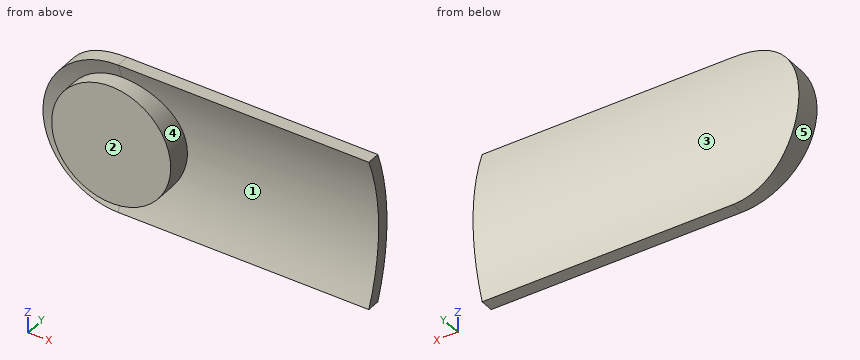
from build123d import *

# Parameters (mm, degrees)
F0_R     = 60.325
F1_DEPTH = 19.05
F4_ANGLE = -180
F2_R     = 203.2
F5_DEPTH = 492.64856
F6_DEPTH = 285.85777
F7_DEPTH = 25.4


with BuildPart() as f1:
    # F0 (on Front) → F1 (new body, symmetric)
    with BuildSketch(Plane.XZ):
        with BuildLine():
            Line((254, 76.2), (0, 76.2))
            ThreePointArc((0, 76.2), (-76.2, 0), (0, -76.2))
            Line((0, -76.2), (254, -76.2))
            Line((254, -76.2), (254, 76.2))
        make_face()
        Circle(F0_R, mode=Mode.SUBTRACT)
        Circle(F0_R)
    extrude(amount=F1_DEPTH, both=True)

    # F3 (on face) → F4 (revolve, cut)
    with BuildSketch(Plane.YZ):
        with BuildLine():
            Line((-406.4, 0), (0, 0))
            ThreePointArc((0, 0), (-203.2, 203.2), (-406.4, 0))
        make_face()
    revolve(axis=Axis((0, -203.2, 0), (0, 1, 0)), revolution_arc=F4_ANGLE, mode=Mode.SUBTRACT)

    # F2 (on Right) → F5 (cut)
    with BuildSketch(Plane.YZ):
        with Locations((-203.2, 0)):
            Circle(F2_R)
    extrude(amount=F5_DEPTH, mode=Mode.SUBTRACT)

    # F2 (on Right) → F6 (cut, symmetric)
    with BuildSketch(Plane.YZ):
        with BuildLine():
            ThreePointArc((-13.238437, 102.60319), (12.640691, -5.060247), (-18.255432, -111.392625))
            Line((-18.255432, -111.392625), (114.283874, -111.392625))
            Line((114.283874, -111.392625), (114.283874, 102.60319))
            Line((114.283874, 102.60319), (-13.238437, 102.60319))
        make_face()
    extrude(amount=F6_DEPTH, both=True, mode=Mode.SUBTRACT)

    # F0 (on Front) → F7 (join)
    with BuildSketch(Plane.XZ):
        Circle(F0_R)
    extrude(amount=F7_DEPTH)


solid = f1.part
Build history of the part. All positions in model axes, mm. Face numbers are marked on the shaded views. A direction names the side the tool comes from. Coordinates: 2 decimals unless noted, no trailing zeros. Write each loop counter-clockwise with the first axis right and the second up, starting at its lowest first coordinate (ties: lowest second). Pieces come first, ordered by that corner, then holes.
(1) 3-axis set-ups, long thin cutter, end or side, ignore diameter. For the marked faces 4 and 5: which of +Z, -Z, +X, -X, +Y, -Y reach the whole face in a straight line?
(2) Cut at B-B on x = 39.5. List the corners of the cut face in (y, z), and give its area (3 significant figures).
(3) Pin check, flat tips, straight feed: pin 1 Ø4 at (x, z) = (205.5, 49) entering from +Y; pin 2 Ø2 at (x, z) = (161.5, -38.5) entering from -Y; pin 3 Ø1 at (x, z) = (5.5, -42) entering from +Y. Stop position of each tip, or through.
(4) Mould opens along Z. For the marked faces 1, 2 and 3 say: pulls with the +Z half, pulls with the -Z half, needs draft (parallel to the pull), parting line crosses it, or undercut.
(5) Cut at D-D on x = 196. List the corners of the cut face in (y, z).
(6) Drill centre lines: line 1 (X direction, y = -4, z = 0.5); line 2 (Y direction, x = -45.5, z = 4.5); line 3 (Y direction, x = 27, z = -6). Where is each one in solid material? Low to high.
(7) Cut at C-C on y = -21. List the corners of the cut face in (x, z) (3 decimals), and give its area (3 significant figures).
(8) Cut at A-A on z = 0. List the corners of the cut face in (x, y) (3 decimals).
Working result:
1. face 4: -Y
1. face 5: -X, +Y, -Y
2. outline: (-25.4, -45.59) - (-5.18, -45.59) arc R203.2 cw to (-14.83, -76.2) - (-1.19, -76.2) arc R215.9 ccw to (-1.19, 76.2) - (-14.83, 76.2) arc R203.2 cw to (-5.18, 45.59) - (-25.4, 45.59) - close
2. area: 4,140 mm2
3. pin 1: stops at y = 7.52
3. pin 2: stops at y = -3.88
3. pin 3: stops at y = 8.67
4. face 1: undercut
4. face 2: needs draft
4. face 3: parting line crosses it
5. outline: (-14.83, -76.2) - (-1.19, -76.2) arc R215.9 ccw to (-1.19, 76.2) - (-14.83, 76.2) arc R203.2 cw to start
6. line 1: x = -76.2 to 60.32
6. line 2: y = -25.4 to 12.65
6. line 3: y = -25.4 to 12.62
7. outline: circle Ø120.65 at (0, 0)
7. area: 11,400 mm2
8. outline: (-76.2, -14.829) arc R203.2 cw to (-60.325, -9.161) - (-60.325, -25.4) - (60.325, -25.4) - (60.325, 0) - (254, 0) - (254, 12.7) - (-76.2, 12.7) - close
